Verification items for the finished model (mm, model axes). A direction names the side the tool comes from. Give positions to 0.01 mm unless a question says otherwise; leave off trailing zeros. Order: outer loops, then holes, each group sorted by start corner. A loop starts at its lowest first (then second) coordinate and runs counter-clockwise, first axis right, second up. Notation, with made-up numbers: (-16, 78) -> (16, 78) arc R31 cw to (16, 113) -> close; hole circle Ø6 at (76, -18). An arc over 180 degrees is marked (long way). One line per question, with ' | ' between items. Start each with the question number.
Q1. Go/stop test with a flat-tipped pin: pin 1 (2 mm diameter, centred on x = -57, z = 29, fed in from +Y). Record where the tip stops, or that it passes through.
Q2. Section check A-A on z = 0. Record the cut outline in (x, y).
Q3. Material ranges on probe 1 along X at (y, z) = (-70, 38); probe 2 along Y at (x, z) = (-56, -46); probe 3 along Z at (x, y) = (-61.25, -23), recorded low to high. Write a range as [from, to].
Q4. Mould release check, pull along Y, two halves, no side actions. Record for faces 3 (the cylindrical face through (-58.04, -14.16, 44.93)), 4 (the cylindrical face through (-62.46, -45.98, -52.43)), 5 (the cylindrical face through (-58, -69.5, 45.1)), 6 (the flat face through (-60, -11, 1)): released by +Y, released by -Y, zero draft, split by the parting line, or undercut.
Q5. Section check B-B on y = -30.5. Record the cut outline in (x, z), plus the area to 3 significant figures.
Q6. Access from +Z, -Z, +X, -X, +Y, -Y to the whole of each face (thin tool, end or side, straight path). Record for faces 1 (the flat face through (-63.059, -45, 1)), 2 (the cylindrical face through (-58.04, -15.31, -1.22)).
from build123d import *

# Parameters (mm, degrees)
F1_START = 11
F1_DEPTH = 69
F4_START = 21.75
F3_R     = 2
F4_DEPTH = 4.25
F5_R     = 2
F6_R     = 2


with BuildPart() as f1:
    # F0 (on Front) → F1 (new body)
    with BuildSketch(Plane.XZ.offset(F1_START)):
        Polygon((-59.0593354404, 0), (-59.0593354404, 53), (-63.0593354404, 53), (-63.0593354404, -53), (-59.0593354404, -53), align=None)
    extrude(amount=F1_DEPTH)

    # F3 (on offset) → F4 (join)
    with BuildSketch(Plane.YZ.offset(-81).offset(F4_START)):
        with Locations((-70.4067274928, -46.8843728304)):
            Circle(F3_R)
        with Locations((-70.4067274928, 0)):
            Circle(F3_R)
        with Locations((-70.4067274928, 46.8843728304)):
            Circle(F3_R)
        with Locations((-37.2223369777, 46.8843728304)):
            Circle(F3_R)
        with Locations((-37.2223369777, 0)):
            Circle(F3_R)
        with Locations((-37.2223369777, -46.8843728304)):
            Circle(F3_R)
        with Locations((-13.7270642444, 46.8843728304)):
            Circle(F3_R)
        with Locations((-13.7270642444, 0)):
            Circle(F3_R)
        with Locations((-13.7270642444, -46.8843728304)):
            Circle(F3_R)
    extrude(amount=F4_DEPTH)

    # F5
    f5_edges = [f1.edges().sort_by_distance(p)[0] for p in [
        (-55, -72.406727, 0),
        (-55, -72.406727, 46.884373),
        (-55, -72.406727, -46.884373),
        (-55, -39.222337, -46.884373),
        (-55, -39.222337, 0),
        (-55, -39.222337, 46.884373),
        (-55, -15.727064, 46.884373),
        (-55, -15.727064, 0),
        (-55, -15.727064, -46.884373),
    ]]
    fillet(f5_edges, radius=F5_R)

    # F6
    f6_edges = [f1.edges().sort_by_distance(p)[0] for p in [
        (-63.059335, -45.5, 53),
        (-63.059335, -45.5, -53),
        (-63.059335, -11, 0),
        (-63.059335, -80, 0),
    ]]
    fillet(f6_edges, radius=F6_R)


solid = f1.part
Filled in:
1) pin 1: through
2) outline: (-63.06, -78) arc R2 ccw to (-61.06, -80) -> (-59.06, -80) -> (-59.06, -72.41) -> (-57, -72.41) arc R2 ccw to (-57, -68.41) -> (-59.06, -68.41) -> (-59.06, -39.22) -> (-57, -39.22) arc R2 ccw to (-57, -35.22) -> (-59.06, -35.22) -> (-59.06, -15.73) -> (-57, -15.73) arc R2 ccw to (-57, -11.73) -> (-59.06, -11.73) -> (-59.06, -11) -> (-61.06, -11) arc R2 ccw to (-63.06, -13) -> close
3) probe 1: [-63.06, -59.06] | probe 2: [-71.9, -68.92], [-38.71, -35.73], [-15.22, -12.24] | probe 3: [-52.99, 52.99]
4) face 3: undercut | face 4: zero draft | face 5: undercut | face 6: released by +Y
5) outline: (-63.06, -51) arc R2 ccw to (-61.06, -53) -> (-59.06, -53) -> (-59.06, 53) -> (-61.06, 53) arc R2 ccw to (-63.06, 51) -> close | area: 422 mm²
6) face 1: +Z, -Z, -X, +Y, -Y | face 2: +X
